Part model, mm, in its own coordinate system. Face numbers are marked on the shaded views. Round coordinates to 2 decimals unless told otherwise and drop trailing zeros. Write each loop counter-clockwise with the first axis right and the second up, starting at its lowest first coordinate (ties: lowest second). Pieces come first, ordered by that corner, then holes. Notation, with made-up numbers: M 43.25,44 L 56.25,44 A10 cw 56.25,57 Z; hole C 45.5,68 d3. An arc over 180 degrees is marked long. Answer as a JSON object with one key per item and string values. Group by question number.
1. Band-saw the part on C-C, the plane y = 183.25. Write the cut outline in (x, z), plus the area to 4 significant figures.
2. Drop a flat-ended pin along its axis: pin 1 (4.5 mm diameter, centred on x = -166.56, z = 11.64, fed in from -Y). Give the stop position or say it passes through.
3. Band-saw the part on A-A, the plane x = -174. Write the cut outline in (y, z), plus the area to 3 significant figures.
4. Band-saw the part on B-B, the plane z = 23.75. Write the cut outline in (x, y), plus the area to 3 significant figures.
5. Drill centre lines: line 1 (Y direction, x = -179.5, z = 5.25); line 2 (X direction, y = 183, z = 13.25); line 3 (X direction, y = 174.75, z = 13). Where is each one in solid material? Low to high. Write a range as from..to.
6. Two-plate mould, pull along Y, no slides. Class the marked faces 1, 2 and 3: +Y half, -Y half, draft (parallel to the pull), parting line (faces both ways), or undercut.
7. Band-saw the part on D-D, the plane z = 20. Write the cut outline in (x, y), plus the area to 3 significant figures.
from build123d import *

# Parameters (mm, degrees)
SALIENTE_EXTRUIR1_DEPTH = 3
CROQUIS2_R              = 1.5
SALIENTE_EXTRUIR2_DEPTH = 6
SALIENTE_EXTRUIR3_START = 3
SALIENTE_EXTRUIR3_DEPTH = 3
CORTAR_EXTRUIR1_REACH   = 194.159
CROQUIS4_R              = 2.5


with BuildPart() as part:
    # Croquis1 → Saliente-Extruir1 (new body)
    with BuildSketch(Plane(origin=(0, 175.405960568, 0), x_dir=(-1, 0, 0), z_dir=(0, -1, 0))):
        with BuildLine():
            Line((159.062896708, 2.364392951), (190.062896708, 2.364392951))
            Line((190.062896708, 2.364392951), (190.062896708, -25.635607049))
            Line((190.062896708, -25.635607049), (159.062896708, -25.635607049))
            ThreePointArc((159.062896708, -25.635607049), (156.234469583, -24.464034173), (155.062896708, -21.635607049))
            Line((155.062896708, -21.635607049), (155.062896708, -1.635607049))
            ThreePointArc((155.062896708, -1.635607049), (156.234469583, 1.192820076), (159.062896708, 2.364392951))
        make_face()
    extrude(amount=SALIENTE_EXTRUIR1_DEPTH)

    # Croquis2 → Saliente-Extruir2 (add)
    with BuildSketch(Plane(origin=(0, 175.405960568, 0), x_dir=(1, 0, 0), z_dir=(0, 1, 0))):
        with Locations(Location((-160.062896708, -2.635607049, 0), (0, 0, 90))):
            Circle(CROQUIS2_R)
        with Locations(Location((-160.062896708, -20.635607049, 0), (0, 0, 90))):
            Circle(CROQUIS2_R)
    extrude(amount=SALIENTE_EXTRUIR2_DEPTH)

    # Croquis3 → Saliente-Extruir3 (add)
    with BuildSketch(Plane(origin=(0, 181.405960568, 0), x_dir=(1, 0, 0), z_dir=(0, 1, 0)).offset(SALIENTE_EXTRUIR3_START)):
        with BuildLine():
            Line((-190.062896708, 2.364392951), (-190.062896708, -25.635607049))
            Line((-190.062896708, -25.635607049), (-159.062896708, -25.635607049))
            ThreePointArc((-159.062896708, -25.635607049), (-156.234469583, -24.464034173), (-155.062896708, -21.635607049))
            Line((-155.062896708, -21.635607049), (-155.062896708, -1.635607049))
            ThreePointArc((-155.062896708, -1.635607049), (-156.234469583, 1.192820076), (-159.062896708, 2.364392951))
            Line((-159.062896708, 2.364392951), (-190.062896708, 2.364392951))
        make_face()
    extrude(amount=-SALIENTE_EXTRUIR3_DEPTH)

    # Cortar-Extruir1: up to this face of the body (flat: up to its plane)
    cortar_extruir1_end = Plane(part.part.faces().sort_by_distance((-172.680086606, 172.405960568, 11.635607049))[0])
    # Croquis4 → Cortar-Extruir1 (cut, up to the picked face)
    with BuildSketch(Plane(origin=(0, 184.405960568, 0), x_dir=(1, 0, 0), z_dir=(0, 1, 0)), mode=Mode.PRIVATE) as cortar_extruir1_sk1:
        with Locations(Location((-166.562896708, -11.635607049, 0), (0, 0, 270))):
            Circle(CROQUIS4_R)
    cortar_extruir1_tool1 = split(extrude(cortar_extruir1_sk1.sketch, amount=-CORTAR_EXTRUIR1_REACH, mode=Mode.PRIVATE), bisect_by=cortar_extruir1_end, keep=Keep.BOTH, mode=Mode.PRIVATE)
    add(cortar_extruir1_tool1.solids().sort_by(Axis((-166.562897, 184.405961, 11.635607), (0, -1, 0)))[0], mode=Mode.SUBTRACT)


solid = part.part
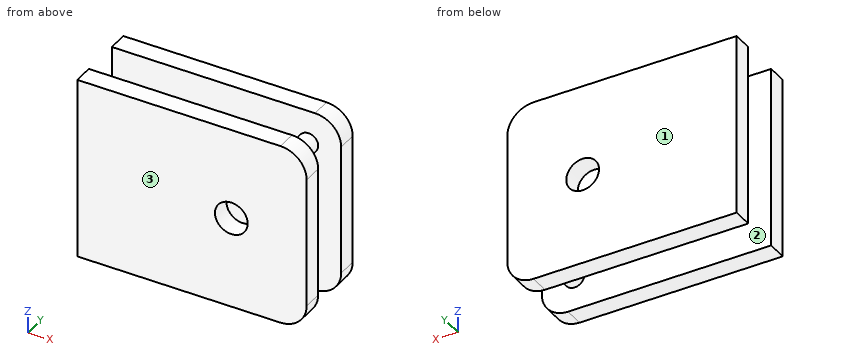
Worked answers:
{
 "1": {"outline": "M -190.06,-2.36 L -159.06,-2.36 A4 ccw -155.06,1.64 L -155.06,21.64 A4 ccw -159.06,25.64 L -190.06,25.64 Z; hole C -166.56,11.64 d5", "area": "953.5 mm^2"},
 "2": {"pin 1": "passes through"},
 "3": {"outline": "M 172.41,-2.36 L 175.41,-2.36 L 175.41,25.64 L 172.41,25.64 Z; M 181.41,-2.36 L 184.41,-2.36 L 184.41,25.64 L 181.41,25.64 Z", "area": "168 mm^2"},
 "4": {"outline": "M -190.06,172.41 L -155.67,172.41 L -155.67,175.41 L -190.06,175.41 Z; M -190.06,181.41 L -155.67,181.41 L -155.67,184.41 L -190.06,184.41 Z", "area": "206 mm^2"},
 "5": {"line 1": "y = 172.41..175.41, 181.41..184.41", "line 2": "x = -190.06..-168.47, -164.65..-155.06", "line 3": "x = -190.06..-168.66, -164.47..-155.06"},
 "6": {"face 1": "+Y half", "face 2": "undercut", "face 3": "-Y half"},
 "7": {"outline": "M -190.06,172.41 L -155.06,172.41 L -155.06,175.41 L -158.7,175.41 L -158.7,181.41 L -155.06,181.41 L -155.06,184.41 L -190.06,184.41 L -190.06,181.41 L -161.42,181.41 L -161.42,175.41 L -190.06,175.41 Z", "area": "226 mm^2"}
}
